from build123d import *

# Parameters (mm, degrees)
ESBO_O1_W                = 45
ESBO_O1_H                = 20
RESSALTO_EXTRUS_O1_DEPTH = 1
ESBO_O2_R                = 8.25
RESSALTO_EXTRUS_O2_DEPTH = 12
ESBO_O3_R                = 7
CORTE_EXTRUS_O1_DEPTH    = 0.5
RESSALTO_EXTRUS_O5_DEPTH = 3.5
ESBO_O7_W                = 1.9
ESBO_O7_H                = 2
ESBO_O7_W_2              = 1.8
RESSALTO_EXTRUS_O6_DEPTH = 2
ESBO_O9_W                = 10
ESBO_O9_H                = 0.1
CORTE_EXTRUS_O2_DEPTH    = 2
ESBO_O10_W               = 1
ESBO_O10_H               = 1
RESSALTO_EXTRUS_O7_DEPTH = 2
ESBO_O11_W               = 1
ESBO_O11_H               = 1
ESBO_O11_H_2             = 0.967747288
RESSALTO_EXTRUS_O8_DEPTH = 4


with BuildPart() as part:
    # Esboço1 → Ressalto-extrusão1 (new body)
    with BuildSketch(Plane.XY):
        with Locations((22.5, 10)):
            Rectangle(ESBO_O1_W, ESBO_O1_H)
    extrude(amount=RESSALTO_EXTRUS_O1_DEPTH)

    # Esboço2 → Ressalto-extrusão2 (add)
    with BuildSketch(Plane.XY.offset(1)):
        with Locations((9.25, 10)):
            Circle(ESBO_O2_R)
        with Locations((35.75, 10)):
            Circle(ESBO_O2_R)
    extrude(amount=RESSALTO_EXTRUS_O2_DEPTH)

    # Esboço3 → Corte-extrusão1 (cut)
    with BuildSketch(Plane.XY.offset(13)):
        with Locations((9.25, 10)):
            Circle(ESBO_O3_R)
        with Locations((35.75, 10)):
            Circle(ESBO_O3_R)
    extrude(amount=-CORTE_EXTRUS_O1_DEPTH, mode=Mode.SUBTRACT)

    # Esboço6 → Ressalto-extrusão5 (add)
    with BuildSketch(Plane.XY.offset(1)):
        with BuildLine():
            Line((25.75, 17.816758405), (19.25, 17.816758405))
            ThreePointArc((19.25, 17.816758405), (17.5, 16.066758405), (19.25, 14.316758405))
            Line((19.25, 14.316758405), (25.75, 14.316758405))
            ThreePointArc((25.75, 14.316758405), (27.5, 16.066758405), (25.75, 17.816758405))
        make_face()
    extrude(amount=RESSALTO_EXTRUS_O5_DEPTH)

    # Esboço7 → Ressalto-extrusão6 (add)
    with BuildSketch(Plane(origin=(0, 0, 0), x_dir=(-1, 0, 0), z_dir=(0, 0, -1))):
        with Locations((-26.55, 1)):
            Rectangle(ESBO_O7_W, ESBO_O7_H)
        with Locations((-24.5, 1)):
            Rectangle(ESBO_O7_W_2, ESBO_O7_H)
        with Locations((-22.5, 1)):
            Rectangle(ESBO_O7_W_2, ESBO_O7_H)
        with Locations((-20.5, 1)):
            Rectangle(ESBO_O7_W_2, ESBO_O7_H)
        with Locations((-18.45, 1)):
            Rectangle(ESBO_O7_W, ESBO_O7_H)
    extrude(amount=RESSALTO_EXTRUS_O6_DEPTH)

    # Esboço9 → Corte-extrusão2 (cut)
    with BuildSketch(Plane(origin=(0, 0, -2), x_dir=(-1, 0, 0), z_dir=(0, 0, -1))):
        with Locations((-22.5, 0.05)):
            Rectangle(ESBO_O9_W, ESBO_O9_H)
    extrude(amount=-CORTE_EXTRUS_O2_DEPTH, mode=Mode.SUBTRACT)

    # Esboço10 → Ressalto-extrusão7 (add)
    with BuildSketch(Plane(origin=(0, 0, -2), x_dir=(-1, 0, 0), z_dir=(0, 0, -1))):
        with Locations((-24.5, 1.05)):
            Rectangle(ESBO_O10_W, ESBO_O10_H)
        with Locations((-26.55, 1.05)):
            Rectangle(ESBO_O10_W, ESBO_O10_H)
        with Locations((-22.472435469, 1.05)):
            Rectangle(ESBO_O10_W, ESBO_O10_H)
        with Locations((-20.46939422, 1.05)):
            Rectangle(ESBO_O10_W, ESBO_O10_H)
        with Locations((-18.471440092, 1.05)):
            Rectangle(ESBO_O10_W, ESBO_O10_H)
    extrude(amount=RESSALTO_EXTRUS_O7_DEPTH)

    # Esboço11 → Ressalto-extrusão8 (add)
    with BuildSketch(Plane.XZ.offset(-0.55)):
        with Locations((26.55, -3.5)):
            Rectangle(ESBO_O11_W, ESBO_O11_H)
        with Locations((24.5, -3.5)):
            Rectangle(ESBO_O11_W, ESBO_O11_H)
        with Locations((22.472435469, -3.516126356)):
            Rectangle(ESBO_O11_W, ESBO_O11_H_2)
        with Locations((20.46939422, -3.516126356)):
            Rectangle(ESBO_O11_W, ESBO_O11_H_2)
        with Locations((18.471440092, -3.516126356)):
            Rectangle(ESBO_O11_W, ESBO_O11_H_2)
    extrude(amount=RESSALTO_EXTRUS_O8_DEPTH)


solid = part.part
Work out the finished part from the listing and answer in its coordinate system (mm). A direction names the side the tool comes from. Round coordinates to 2 decimals unless told otherwise and drop trailing zeros. Write each loop counter-clockwise with the first axis right and the second up, starting at its lowest first coordinate (ties: lowest second). Pieces come first, ordered by that corner, then holes. Notation, with made-up numbers: (-12.5, 26) -> (43.5, 26) arc R20 ccw to (43.5, 41) -> close; hole circle Ø8 at (55.5, 52.5). An arc over 180 degrees is marked (long way). Answer as CSV lines item,"result". Start each with the question number.
(1) The part is cut by section A-A, the plane z = -2.5. Give the vertices of the cut face in (x, y).
(2) The mould has two halves that part along Z. Classify faces 4 (the flat face through (26.5, -0.9, -4)), 5 (the flat face through (26.6, 0.4, -2)), 6 (the flat face through (22.2, 20, 0.5)): +Z half, -Z half, draft (parallel to the pull), parting line (faces both ways), or undercut.
(3) The part is cut by section D-D, the plane x = 35.75. Give the vertices of the cut face in (y, z), then the cut area to 3 significant figures.
(4) A tool of negligible diameter and unlimited length cuts with its end or side. For faces 1 (the flat face through (9, 10, 12.5)), 2 (the flat face through (21, 2, -1)), 3 (the flat face through (26.05, -0.4, -3.2)), from which of +Z, -Z, +X, -X, +Y, -Y can it reach the whole face along a straight path? Write none if from no direction.
(5) Each of these flat-tipped pins is pushed along its axis until it touches: pin 1 (0.6 mm diameter, centred on y = 0, z = -3.5, fed in from +X); pin 2 (1 mm diameter, centred on y = 1.5, z = -1.5, fed in from +X); pin 3 (2 mm diameter, centred on y = -0.5, z = -3.5, fed in from -X); pin 4 (5 mm diameter, centred on x = 29, y = 16, fed in from +Z). Where does it stop, or does it pass through?
(6) The part is cut by section C-C, the plane z = 2.75. Give the vertices of the cut face in (x, y).
(7) The part is cut by section B-B, the plane y = 10. Give the vertices of the cut face in (x, z), then the cut area to 3 significant figures.
(8) Find the intervals of material crossed by probe 1 along Y at (x, z) = (35.75, 12.9); probe 2 along X at (y, z) = (15.5, 2); probe 3 along Z at (x, y) = (10, 12.5), in increasing order.
Output values:
1,outline,"(17.97, 0.55) -> (18.97, 0.55) -> (18.97, 1.55) -> (17.97, 1.55) -> close; (19.97, 0.55) -> (20.97, 0.55) -> (20.97, 1.55) -> (19.97, 1.55) -> close; (21.97, 0.55) -> (22.97, 0.55) -> (22.97, 1.55) -> (21.97, 1.55) -> close; (24, 0.55) -> (25, 0.55) -> (25, 1.55) -> (24, 1.55) -> close; (26.05, 0.55) -> (27.05, 0.55) -> (27.05, 1.55) -> (26.05, 1.55) -> close"
2,face 4,"-Z half"
2,face 5,"undercut"
2,face 6,"draft"
3,outline,"(0, 0) -> (20, 0) -> (20, 1) -> (18.25, 1) -> (18.25, 13) -> (17, 13) -> (17, 12.5) -> (3, 12.5) -> (3, 13) -> (1.75, 13) -> (1.75, 1) -> (0, 1) -> close"
3,area,"211 mm²"
4,face 1,"+Z"
4,face 2,"-Z, +X, -X, +Y"
4,face 3,"-Z, +Y, -Y"
5,pin 1,"stops at x = 27.05"
5,pin 2,"stops at x = 27.5"
5,pin 3,"stops at x = 17.97"
5,pin 4,"stops at z = 13"
6,outline,"circle Ø16.5 at (9.25, 10); (19.25, 14.32) -> (25.75, 14.32) arc R1.75 ccw to (25.75, 17.82) -> (19.25, 17.82) arc R1.75 ccw to start; circle Ø16.5 at (35.75, 10)"
7,outline,"(0, 0) -> (45, 0) -> (45, 1) -> (44, 1) -> (44, 13) -> (42.75, 13) -> (42.75, 12.5) -> (28.75, 12.5) -> (28.75, 13) -> (27.5, 13) -> (27.5, 1) -> (17.5, 1) -> (17.5, 13) -> (16.25, 13) -> (16.25, 12.5) -> (2.25, 12.5) -> (2.25, 13) -> (1, 13) -> (1, 1) -> (0, 1) -> close"
7,area,"427 mm²"
8,probe 1,"y = 1.75 to 3, 17 to 18.25"
8,probe 2,"x = 3.1 to 15.4, 17.59 to 27.41, 29.6 to 41.9"
8,probe 3,"z = 0 to 12.5"
